Geometry check sheet. Reference: drawing and pictorial views, mm from the part's lowest x, y, z. Round coordinates to 2 decimals unless told otherwise and drop trailing zeros. Write each loop counter-clockwise with the first axis right and the second up, starting at its lowest first coordinate (ties: lowest second). Pieces come first, ordered by that corner, then holes. Notation, with made-up numbers: M 56.25,40.5 L 81.25,40.5 A21 ccw 81.25,70.5 Z; hole C 9.25,60 d11. An arc over 180 degrees is marked long. Use a Markdown table: item, result. Add a question column.
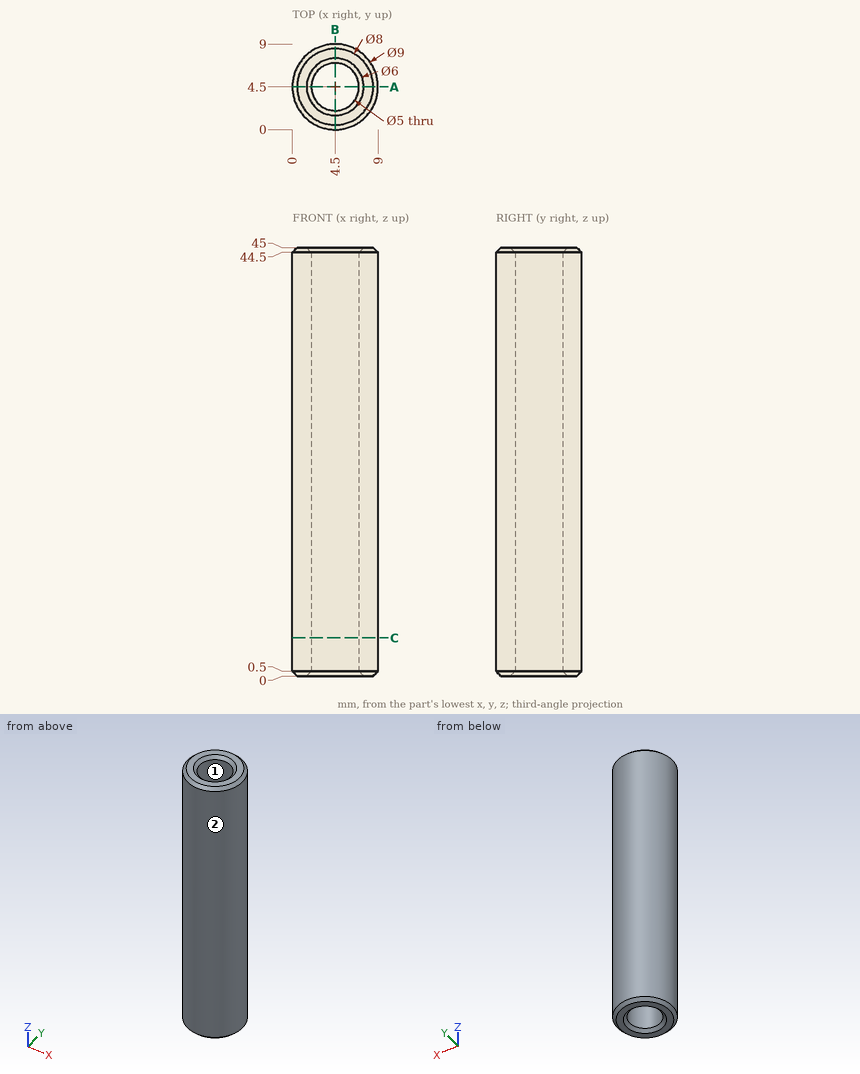
1. Cross-section at A-A on y = 4.5. Enter the section's corners in (x, z), plus the area to 3 significant figures.
2. Depth check by flat-ended pin: pin 1 Ø1.5 at (x, y) = (5.5, 6) entering from +Z; pin 2 Ø2 at (x, z) = (3, 8) entering from -Y; pin 3 Ø1.5 at (x, z) = (7.5, 29) entering from -Y. Enter the tip coordinate at first touch or a pass-through.
3. Scan lines: line 1 along Y through (x, z) = (4.5, 14.5); line 2 along X through (y, z) = (3, 9.5); line 3 along X through (y, z) = (5.5, 20). Record each from-to range of solid material in increasing order. Write a range as from..to.
4. Cross-section at C-C on z = 4. Enter the section's corners in (x, y).
5. Release check for a two-part mould opening along Y. For the marked faces 1 and 2 record: +Y half, -Y half, draft (parallel to the pull), parting line (faces both ways), or undercut.
Answer:
| question | item | result |
|---|---|---|
| 1 | outline | M 0,0.5 L 0.5,0 L 1.5,0 L 2,0.5 L 2,44.5 L 1.5,45 L 0.5,45 L 0,44.5 Z; M 7,0.5 L 7.5,0 L 8.5,0 L 9,0.5 L 9,44.5 L 8.5,45 L 7.5,45 L 7,44.5 Z |
| 1 | area | 179 mm^2 |
| 2 | pin 1 | stops at z = 44.55 |
| 2 | pin 2 | stops at y = 0.03 |
| 2 | pin 3 | stops at y = 0.6 |
| 3 | line 1 | y = 0..2, 7..9 |
| 3 | line 2 | x = 0.26..2.5, 6.5..8.74 |
| 3 | line 3 | x = 0.11..2.21, 6.79..8.89 |
| 4 | outline | C 4.5,4.5 d9; hole C 4.5,4.5 d5 |
| 5 | face 1 | undercut |
| 5 | face 2 | parting line |
